Work out the finished part from the listing and answer in its coordinate system (mm). A direction names the side the tool comes from. Round coordinates to 2 decimals unless told otherwise and drop trailing zeros. Order: outer loops, then holes, each group sorted by start corner. A loop starts at its lowest first (then second) coordinate and runs counter-clockwise, first axis right, second up. Notation, with made-up numbers: (-12, 30) - (41, 30) arc R31 ccw to (41, 55) - close; hole circle Ø8 at (51.25, 4.5). An arc over 180 degrees is marked (long way). Use CSV: the item, a comma, the result in double quotes.
from build123d import *

# Parameters (mm, degrees)
BOSS_EXTRUDE1_DEPTH      = 120
BOSS_EXTRUDE1_DEPTH_BACK = 90
SKETCH1_R                = 24.75
SKETCH1_R_2              = 21.75
BOSS_EXTRUDE3_START      = 72
SKETCH5_R                = 29.75
SKETCH5_R_2              = 21.75
BOSS_EXTRUDE3_DEPTH      = 5
SKETCH7_R                = 24.75
SKETCH7_R_2              = 21.75
BOSS_EXTRUDE4_DEPTH      = 2.5
BOSS_EXTRUDE5_START      = -5
SKETCH6_R                = 2
BOSS_EXTRUDE5_DEPTH      = 5
MIRROR2_START            = 67
MIRROR2_OUTLINE_R        = 29.75
MIRROR2_OUTLINE_R_2      = 24.75
MIRROR2_DEPTH            = 5
MIRROR2_START_2          = -90
MIRROR2_2_OUTLINE_R      = 2
MIRROR2_2_DEPTH          = 5


# Read off the part's stored shape, not the designer's step: Mirror2
with BuildPart() as part:
    # Sketch1 → Boss-Extrude1 (new, two sides: drawn at the far end of the back side and taken through both)
    with BuildSketch(Plane.XY.offset(-BOSS_EXTRUDE1_DEPTH_BACK)):
        Circle(SKETCH1_R)
        Circle(SKETCH1_R_2, mode=Mode.SUBTRACT)
    extrude(amount=BOSS_EXTRUDE1_DEPTH + BOSS_EXTRUDE1_DEPTH_BACK)

    # Sketch5 → Boss-Extrude3 (add)
    with BuildSketch(Plane.XY.offset(BOSS_EXTRUDE3_START)):
        Circle(SKETCH5_R)
        Circle(SKETCH5_R_2, mode=Mode.SUBTRACT)
    extrude(amount=BOSS_EXTRUDE3_DEPTH)

    # Sketch7 → Boss-Extrude4 (add, symmetric)
    with BuildSketch(Plane.XY.offset(120)):
        Circle(SKETCH7_R)
        Circle(SKETCH7_R_2, mode=Mode.SUBTRACT)
    extrude(amount=BOSS_EXTRUDE4_DEPTH, both=True)

    # Sketch6 → Boss-Extrude5 (add)
    with BuildSketch(Plane.XY.offset(122.5).offset(BOSS_EXTRUDE5_START)):
        with BuildLine():
            Line((-22.997666259, 9.147122314), (-33.267406372, 22.947582732))
            Line((-33.267406372, 22.947582732), (-22.947582732, 33.267406372))
            Line((-22.947582732, 33.267406372), (-9.147122314, 22.997666259))
            ThreePointArc((-9.147122314, 22.997666259), (-17.500892834, 17.500892834), (-22.997666259, 9.147122314))
        make_face()
        with Locations((-20.04683438, 22.097086912)):
            Circle(SKETCH6_R, mode=Mode.SUBTRACT)
        with Locations((-27.04683438, 22.097086912)):
            Circle(SKETCH6_R, mode=Mode.SUBTRACT)
    boss_extrude5 = extrude(amount=BOSS_EXTRUDE5_DEPTH)

    # Mirror1: Boss-Extrude5 across plane
    add(boss_extrude5.mirror(Plane(origin=(0, 0, 0), x_dir=(0, 0, 1), z_dir=(1, 0, 0))))

    # Mirror2 outline → Mirror2 (add)
    with BuildSketch(Plane.XY.offset(MIRROR2_START)):
        Circle(MIRROR2_OUTLINE_R)
        Circle(MIRROR2_OUTLINE_R_2, mode=Mode.SUBTRACT)
    extrude(amount=MIRROR2_DEPTH)

    # Mirror2 2 outline → Mirror2 2 (add)
    # profile 1 of 2: a face of its own
    with BuildSketch(Plane.XY.offset(MIRROR2_START_2)):
        with BuildLine():
            Line((22.997666259, 9.147122314), (33.267406372, 22.947582732))
            Line((33.267406372, 22.947582732), (22.947582732, 33.267406372))
            Line((22.947582732, 33.267406372), (9.147122314, 22.997666259))
            ThreePointArc((9.147122314, 22.997666259), (17.500892834, 17.500892834), (22.997666259, 9.147122314))
        make_face()
        with Locations((20.04683438, 22.097086912)):
            Circle(MIRROR2_2_OUTLINE_R, mode=Mode.SUBTRACT)
        with Locations((27.04683438, 22.097086912)):
            Circle(MIRROR2_2_OUTLINE_R, mode=Mode.SUBTRACT)
    # profile 2 of 2: a face of its own
    with BuildSketch(Plane.XY.offset(MIRROR2_START_2)):
        with BuildLine():
            Line((-33.267406372, 22.947582732), (-22.997666259, 9.147122314))
            ThreePointArc((-22.997666259, 9.147122314), (-17.500892834, 17.500892834), (-9.147122314, 22.997666259))
            Line((-9.147122314, 22.997666259), (-22.947582732, 33.267406372))
            Line((-22.947582732, 33.267406372), (-33.267406372, 22.947582732))
        make_face()
        with Locations((-20.04683438, 22.097086912)):
            Circle(MIRROR2_2_OUTLINE_R, mode=Mode.SUBTRACT)
        with Locations((-27.04683438, 22.097086912)):
            Circle(MIRROR2_2_OUTLINE_R, mode=Mode.SUBTRACT)
    extrude(amount=MIRROR2_2_DEPTH)


solid = part.part
(1) The mould has two halves that part along Y. Classify faces 1 (the cylindrical face through (21.634, 20.88, 119.965)), 2 (the flat face through (0, 24, -90)), 3 (the flat face through (-28.18, 28.035, 119.965)): released by +Y, released by -Y, zero draft, split by the parting line, or undercut.
Findings below:
face 1,"undercut"
face 2,"zero draft"
face 3,"released by +Y"
(2) Find the intervals of material crossed by L1, parallel to Z at x = 15, y = 25; L2, parallel to Y at x = -1, z = -69.5; L3, parallel to Y at x = -19, z = -7, in increasing order. Write a range as from..to.
Findings below:
L1,"z = -90..-85, 67..77, 117.5..122.5"
L2,"y = -24.73..-21.73, 21.73..24.73"
L3,"y = -15.86..-10.59, 10.59..15.86"
(3) Each of these flat-tipped pins is pushed along its axis until it touches: pin 1 (6 mm diameter, centred on x = 20, z = -20, fed in from -Y); pin 2 (3.5 mm diameter, centred on x = -27.05, y = 22.1, fed in from -Z); pin 3 (8 mm diameter, centred on x = 13, z = 98, fed in from +Y); pin 4 (4 mm diameter, centred on x = 1, z = -35.5, fed in from -Y). Where does it stop, or does it pass through?
Findings below:
pin 1,"stops at y = -17.99"
pin 2,"passes through"
pin 3,"stops at y = 23.06"
pin 4,"stops at y = -24.75"
(4) Find section A-A (y = 0). Determine the outline of the cut face in (x, z).
Findings below:
outline,"(-29.75, 67) - (-24.75, 67) - (-24.75, -90) - (-21.75, -90) - (-21.75, 122.5) - (-24.75, 122.5) - (-24.75, 77) - (-29.75, 77) - close; (21.75, -90) - (24.75, -90) - (24.75, 67) - (29.75, 67) - (29.75, 77) - (24.75, 77) - (24.75, 122.5) - (21.75, 122.5) - close"
(5) Find section C-C (z = 29). Determine the outline of the cut face in (x, y).
Findings below:
outline,"circle Ø49.5 at (0, 0); hole circle Ø43.5 at (0, 0)"
(6) Find section D-D (x = -14). Determine the outline of the cut face in (y, z), and give its area (3 significant figures).
Findings below:
outline,"(-26.25, 67) - (-20.41, 67) - (-20.41, -90) - (-16.65, -90) - (-16.65, 122.5) - (-20.41, 122.5) - (-20.41, 77) - (-26.25, 77) - close; (16.65, -90) - (26.61, -90) - (26.61, -85) - (20.41, -85) - (20.41, 67) - (26.25, 67) - (26.25, 77) - (20.41, 77) - (20.41, 117.5) - (26.61, 117.5) - (26.61, 122.5) - (16.65, 122.5) - close"
area,"1,780 mm²"
(7) For faces 4 (the flat face through (24, 21, 117.5)), 5 (the flat face through (28.06, 15.95, 119.96)), 6 (the flat face through (16.14, 28.2, 119.96)), 7 (the flat face through (-24.4, -6.5, 77)), 8 (the flat face through (28.06, 15.95, -87.54)), determine the directions among +Z, -Z, +X, -X, +Y, -Y from which every point of the face is accessible in a straight line to the end or side of a thin tool.
Findings below:
face 4,"+X, +Y"
face 5,"+Z, +X"
face 6,"+Z, +Y"
face 7,"none"
face 8,"-Z, +X"
